Autodesk Inventor part; units mm, degrees
ref_plane "Work Plane2" through (3.35, 0, 0) normal (0, 0, -1) x (1, 0, 0)
ref_plane "YZ Plane" through (0, 0, 0) normal (1, 0, 0) x (0, 1, 0)
ref_plane "XZ Plane" through (0, 0, 0) normal (0, 1, 0) x (-1, 0, 0)
sketch "Sketch1" plane through (0, 0, 0) normal (0, 0, 1) x (1, 0, 0)
  line L0 (2.1, 0) -> (12, 0)
  line L1 (12, 0) -> (12, 1.5)
  line L2 (12, 1.5) -> (2.65, 1.5)
  line L3 (2.65, 1.5) -> (2.3433, 1.3466)
  line L4 (2.3433, 1.3466) -> (1.65, 1.3466)
  line L5 (0, 2.75) -> (0, 1.6)
  line L6 (0, 1.6) -> (1.6999, 0.7525)
  line L7 (1.6999, 0.7525) -> (2.1, 0)
  line L8 (-2.4, 0) -> (14.4, 0)
  line L9 (0, -0.55) -> (0, 3.3)
  line L10 (0, 2.75) -> (0.2466, 2.75)
  line L11 (0.2466, 2.75) -> (1.65, 1.3466)
  line L12 (2.65, 1.5) -> (1.4966, 1.5) construction
  dimension "d1" = 9.35
  dimension "d2" = 3
  dimension "d3" = 2.6933
  dimension "d4" = 3.2
  dimension "d5" = 26.5
  dimension "d6" = 62
  dimension "d7" = 2.1
  dimension "d8" = 0.3067
  dimension "d12" = 5.5
  dimension "d13" = 45
  dimension "d15" = 12
  dimension "d24" = 1.65
revolve "Body" add sketch "Sketch1" angle 360 about axis through (2.1, 0, 0) along (1, 0, 0) contours L7 L6 L5 L10 L11 L4 L3 L2 L1 L0
sketch "Sketch2" plane through (0, 0, 0) normal (-1, 0, 0) x (0, 0, 1)
  line L0 (0, 1.6) -> (0, 0) construction
  line L1 (0, 0) -> (1.6, 0) construction
  arc A0 (0.48, 0) -> (0, 0.48) centre (0, 0) ccw construction
  arc A1 (0.56, 0) -> (0, 0.56) centre (0, 0) ccw construction
  arc A2 (1.5795, 0.255) -> (0.255, 1.5795) centre (0, 0) ccw
  line L2 (0, 0) -> (1.1314, 1.1314) construction
  line L3 (0.255, 1.5795) -> (0.2766, 0.4869)
  line L4 (1.5795, 0.255) -> (0.4869, 0.2766)
  arc A3 (0.255, 1.5795) -> (0, 1.6) centre (0, 0) ccw
  arc A4 (1.6, 0) -> (1.5795, 0.255) centre (0, 0) ccw
  line L5 (0, -3.85) -> (0, 3.85)
  line L6 (-3.85, 0) -> (3.85, 0)
  arc A5 (0.255, -1.5795) -> (1.5795, -0.255) centre (0, 0) ccw
  line L7 (0.255, -1.5795) -> (0.2766, -0.4869)
  line L8 (1.5795, -0.255) -> (0.4869, -0.2766)
  arc A6 (0, -1.6) -> (0.255, -1.5795) centre (0, 0) ccw
  arc A7 (1.5795, -0.255) -> (1.6, 0) centre (0, 0) ccw
  arc A8 (-0.255, 1.5795) -> (-1.5795, 0.255) centre (0, 0) ccw
  line L9 (-0.255, 1.5795) -> (-0.2766, 0.4869)
  line L10 (-1.5795, 0.255) -> (-0.4869, 0.2766)
  arc A9 (0, 1.6) -> (-0.255, 1.5795) centre (0, 0) ccw
  arc A10 (-1.5795, 0.255) -> (-1.6, 0) centre (0, 0) ccw
  arc A11 (-0.255, -1.5795) -> (0, -1.6) centre (0, 0) ccw
  arc A12 (-1.5795, -0.255) -> (-0.255, -1.5795) centre (0, 0) ccw
  arc A13 (-1.6, 0) -> (-1.5795, -0.255) centre (0, 0) ccw
  line L11 (-1.5795, -0.255) -> (-0.4869, -0.2766)
  line L12 (-0.255, -1.5795) -> (-0.2766, -0.4869)
  arc A14 (0.2766, 0.4869) -> (0.4869, 0.2766) centre (0.4912, 0.4912) ccw
  arc A15 (0.4869, -0.2766) -> (0.2766, -0.4869) centre (0.4912, -0.4912) ccw
  arc A16 (-0.4869, 0.2766) -> (-0.2766, 0.4869) centre (-0.4912, 0.4912) ccw
  arc A17 (-0.2766, -0.4869) -> (-0.4869, -0.2766) centre (-0.4912, -0.4912) ccw
  point P0 (1.1314, -1.1314)
  point P1 (-1.1314, 1.1314)
  point P2 (-1.1314, -1.1314)
  dimension "d17" = 0.96
  dimension "d18" = 1.12
  dimension "d19" = 3.2
  dimension "d20" = 45
  dimension "d21" = 0.255
extrude "Slot" add sketch "Sketch2" against normal up to next draft 5 contours L4 A14 L3 A2 | A5 L7 A15 L8 | L9 A16 L10 A8 | A12 L11 A17 L12
fillet "Fillet1" radius 0.102 4 edges at (0, 1.6, 0) (0, 0, -1.6) (0, -1.6, 0) (0, 0, 1.6)
thread "Thread"
chamfer "Chamfer1" distance 0.3067 distance2 0.1534 1 edges at (12, -1.5, 0) measured on face at (12, 0.263, 0.1197)
ref_plane "Work Plane2" through (3.35, 0, 0) normal (0, 0, -1) x (1, 0, 0)
equation "\"d1\" = GEL"
equation "\"d2\" = GD"
equation "\"d3\" = BDM"
equation "\"d4\" = SDM"
equation "\"d7\" = INTI"
equation "\"d8\" = GAL"
equation "\"d12\" = KOD"
equation "\"d13\" = 0.5 * SEWI"
equation "\"d15\" = NLG"
equation "\"d24\" = KOH"
equation "\"d17\" = 0.3 * SDM"
equation "\"d18\" = 0.35 * SDM"
equation "\"d19\" = SDM"
equation "\"d21\" = 0.5 * SBR"
equation "\"d23\" = 0.2 * SBR"
equation "\"d10\" = GEL"
equation "\"d25\" = -0.5 * SPD + 0.5 * GD"
equation "\"d26\" = 0.5 * GAL"
equation "\"NLG\" = 12"
equation "\"GEL\" = 9.35"
equation "\"GAL\" = 0.61345 * PTC"
equation "\"SPD\" = NND - 1.2269 * PTC"
equation "\"KOD\" = 5.5"
equation "\"KOH\" = 1.65"
equation "\"SBR\" = 0.51"
equation "\"INTI\" = 2.1"
equation "\"SDM\" = 3.2"
equation "\"GD\" = NND"
equation "\"BDM\" = NND - GAL"
equation "\"SEWI\" = 90deg"
equation "\"d9\" = SDM"
equation "\"GUL\" = 0.61345 * PTC"
equation "\"TOA\" = 30deg"
equation "\"EPV\" = 3.15"
equation "\"THREADDIA\" = 3"
equation "\"PTC\" = 0.5"
equation "\"NND\" = 3"
equation "\"GD1\" = THREADDIA - 1.2269 * PTC"
properties part number "ISO 7046-1 - M3 x 12 - 4.8 - H" material "Steel"
Work out the finished part from the listing and answer in its coordinate system (mm). A direction names the side the tool comes from. Give positions to 0.01 mm unless a question says otherwise; leave off trailing zeros. Loops run counter-clockwise (first coordinate to the right, second up) from the corner with the lowest first, then second, coordinate; pieces in that order, holes last. Notation, with made-up numbers: (-27.75, 48.25) - (24.25, 48.25) arc R23 cw to (24.25, 69.25) - close; hole circle Ø7 at (64.25, 27). An arc over 180 degrees is marked (long way). Answer in a Markdown table with one row per item. Add a question column.
Q1. A tool of negligible diameter and unlimited length cuts with its end or side. For faces 4 (the cylindrical face through (7.18, -1.5, -0.07)), 5 (the conical face through (0.867, 0.003, -1.168)), from which of +Z, -Z, +X, -X, +Y, -Y can it reach the whole face along a straight path? Write none if from no direction.
Q2. Consider line 1 along Z through (x, y) = (6.25, 0); line 2 along X through (y, z) = (0.85, -0.05); line 3 along Y through (x, z) = (11, 1.1). Determine where each line is inside the solid, lowest interval first.
Q3. Each of these flat-tipped pins is pushed along its axis until it touches: P1, Ø3, axis at x = 5, y = -2, coming from the -Z side; P2, Ø1.5, axis at x = 6, y = 2, coming from the +Z side; P3, Ø3, axis at x = 3, y = -0.5, coming from the -Z side. Where does it stop, or does it pass through?
Q4. Determine the mould class of faces 1 (the cylindrical face through (1.992, -1.345, -0.059)), 2 (the conical face through (0.867, -0.003, 1.168)), 3 (the flat face through (12, 0, 0)) for opening direction Y: released by +Y, released by -Y, zero draft, split by the parting line, or undercut.
Q5. The part is cut by section A-A (x = 3). Determine the outline of the cut face in (y, z), and give its area (3 significant figures).
Solution:
| question | item | result |
|---|---|---|
| 1 | face 4 | +X |
| 1 | face 5 | -X |
| 2 | line 1 | z = -1.5 to 1.5 |
| 2 | line 2 | x = 1.5 to 12 |
| 2 | line 3 | y = -1.02 to 1.02 |
| 3 | P1 | stops at z = -1.41 |
| 3 | P2 | stops at z = 0.83 |
| 3 | P3 | stops at z = -1.5 |
| 4 | face 1 | split by the parting line |
| 4 | face 2 | undercut |
| 4 | face 3 | zero draft |
| 5 | outline | circle Ø3 at (0, 0) |
| 5 | area | 7.07 mm² |
